The model under review builds one solid part; all positions refer to its coordinate system, in mm. A direction names the side the tool comes from. Coordinates: 2 decimals unless noted, no trailing zeros. Write each loop counter-clockwise with the first axis right and the second up, starting at its lowest first coordinate (ties: lowest second). Pieces come first, ordered by that corner, then holes. Notation, with made-up numbers: (-29.5, 71.5) - (-18.5, 71.5) arc R27 cw to (-18.5, 107.5) - close; hole circle Ø4 at (-32, 10). An arc over 180 degrees is marked (long way). Return JSON: item names as keys, results as strings. Group by question number.
(1) Draft analysis for pull direction X (two halves, no side actions). For faces 1 (the face through (-39.365, 61.689, -0.133)), 2 (the face through (61, -25, 61.925)), 3 (the face through (63.867, -25, 41)), 4 (the face through (114.667, -25, 52)), state which applies: released by +X, released by -X, zero draft, split by the parting line, or undercut.
(2) Tool access review of faces 5 (the face through (89, -25, 38.1)), 6 (the face through (68, -50.8, 45)), 7 (the face through (22.225, -33, 18)): name each direction out of +Z, -Z, +X, -X, +Y, -Y from which nothing blocks a thin tool from reaching the whole face with its end or side.
(3) To check wall thickness, follow L1, parallel to X at y = -31, z = -3 (3 decimals); L2, parallel to Z at x = 6, y = 33.5 (3 decimals); L3, parallel to Y at x = 89.5, z = 53.5. State the ranges of each line that lie inside material, in increasing order. Write a range as from..to.
(4) We need section B-B on z = -1.5. State the section outline as (x, y) points (3 decimals).
(5) For pin 1 Ø3 at (x, z) = (37.5, 41) entering from +Y; pin 2 Ø1 at (x, z) = (41.5, 24.5) entering from -Y; pin 3 Ø11 at (y, z) = (-4.5, 17) entering from +X (3 decimals); pin 4 Ø14 at (y, z) = (-28.5, 16) entering from -X (3 decimals), all flat-tipped, find the tip position at first contact; note any pin that passes through.
(6) We need section C-C on x = 76. State the section outline as (y, z) points (3 decimals), then the cut area to 3 significant figures.
(7) We need section A-A on y = -43.5. State the section outline as (x, z) points (3 decimals).
(8) We need section D-D on y = 43. State the section outline as (x, z) points (3 decimals), then the cut area to 3 significant figures.
```python
from build123d import *

# Parameters (mm, degrees)
F1_DEPTH = 63.5
F2_DEPTH = 50.8
F0_W     = 25.4
F0_H     = 19.05
F0_H_2   = 4.7498004709
F0_H_3   = 4.7751995291
F3_DEPTH = 50.8
F4_DEPTH = 15.875
F5_R     = 6.35


with BuildPart() as f1:
    # F0 (on Front) → F1 (new body, symmetric)
    with BuildSketch(Plane.XZ):
        Polygon((-41.275, 9.525), (-41.275, -9.525), (41.275, -9.525), (41.275, 9.525), (22.225, 9.525), align=None)
    extrude(amount=F1_DEPTH, both=True)

    # F0 (on Front) → F2 (join)
    with BuildSketch(Plane.XZ):
        with BuildLine():
            Line((22.225, 9.525), (41.275, 9.525))
            Line((41.275, 9.525), (41.275, 27.0002))
            ThreePointArc((41.275, 27.0002), (45.9246798487, 38.2255201513), (57.15, 42.8752))
            Line((57.15, 42.8752), (63.8665184379, 42.8752))
            Line((63.8665184379, 42.8752), (63.8665184379, 61.9252))
            Line((63.8665184379, 61.9252), (57.15, 61.9252))
            ThreePointArc((57.15, 61.9252), (32.4542956671, 51.6959043329), (22.225, 27.0002))
            Line((22.225, 27.0002), (22.225, 9.525))
        make_face()
    extrude(amount=F2_DEPTH)

    # F0 (on Front) → F3 (join)
    with BuildSketch(Plane.XZ):
        with Locations((76.5665184379, 52.4002)):
            Rectangle(F0_W, F0_H)
        Polygon((89.2665184379, 66.6750004709), (89.2665184379, 61.9252), (89.2665184379, 42.8752), (89.2665184379, 38.1000004709), (114.6665184379, 38.1000004709), (114.6665184379, 66.6750004709), align=None)
        with Locations((76.5665184379, 64.3001002354)):
            Rectangle(F0_W, F0_H_2)
        with Locations((76.5665184379, 40.4876002354)):
            Rectangle(F0_W, F0_H_3)
    extrude(amount=F3_DEPTH)

    # F0 (on Front) → F4 (join)
    with BuildSketch(Plane.XZ):
        Polygon((-41.275, 9.525), (-41.275, -9.525), (41.275, -9.525), (41.275, 9.525), (22.225, 9.525), align=None)
        with BuildLine():
            add(Edge.make_bspline(
                [(-41.275, 9.525), (-41.1059595644, 38.1653234363), (12.9924593493, 62.6207739115), (57.15, 61.9252)],
                knots=[0, 0, 0, 0, 111.5045361635, 111.5045361635, 111.5045361635, 111.5045361635], degree=3))
            Line((-41.275, 9.525), (22.225, 9.525))
            Line((22.225, 9.525), (22.225, 27.0002))
            ThreePointArc((22.225, 27.0002), (32.4542956671, 51.6959043329), (57.15, 61.9252))
        make_face()
        with BuildLine():
            Line((22.225, 9.525), (41.275, 9.525))
            Line((41.275, 9.525), (41.275, 27.0002))
            ThreePointArc((41.275, 27.0002), (45.9246798487, 38.2255201513), (57.15, 42.8752))
            Line((57.15, 42.8752), (63.8665184379, 42.8752))
            Line((63.8665184379, 42.8752), (63.8665184379, 61.9252))
            Line((63.8665184379, 61.9252), (57.15, 61.9252))
            ThreePointArc((57.15, 61.9252), (32.4542956671, 51.6959043329), (22.225, 27.0002))
            Line((22.225, 27.0002), (22.225, 9.525))
        make_face()
        with Locations((76.5665184379, 52.4002)):
            Rectangle(F0_W, F0_H)
        with Locations((76.5665184379, 64.3001002354)):
            Rectangle(F0_W, F0_H_2)
        with Locations((76.5665184379, 40.4876002354)):
            Rectangle(F0_W, F0_H_3)
        Polygon((89.2665184379, 66.6750004709), (89.2665184379, 61.9252), (89.2665184379, 42.8752), (89.2665184379, 38.1000004709), (114.6665184379, 38.1000004709), (114.6665184379, 66.6750004709), align=None)
    extrude(amount=F4_DEPTH)

    # F5
    f5_edges = [f1.edges().sort_by_distance(p)[0] for p in [
        (41.275, -63.5, 0),
        (-41.275, -63.5, 0),
        (41.275, 63.5, 0),
        (-41.275, 63.5, 0),
    ]]
    fillet(f5_edges, radius=F5_R)


solid = f1.part
```
Ans:
{
 "1": {"face 1": "released by -X", "face 2": "zero draft", "face 3": "undercut", "face 4": "released by +X"},
 "2": {"face 5": "-Z, +X, +Y, -Y", "face 6": "+Z, +X, -X, -Y", "face 7": "+Z, -X, -Y"},
 "3": {"L1": "-41.275..41.275", "L2": "-9.525..9.525", "L3": "-50.8..0"},
 "4": {"outline": "(-41.275, -57.15) arc R6.35 ccw to (-34.925, -63.5) - (34.925, -63.5) arc R6.35 ccw to (41.275, -57.15) - (41.275, 57.15) arc R6.35 ccw to (34.925, 63.5) - (-34.925, 63.5) arc R6.35 ccw to (-41.275, 57.15) - close"},
 "5": {"pin 1": "y = 0", "pin 2": "y = -50.8", "pin 3": "x = 41.275", "pin 4": "x = -41.275"},
 "6": {"outline": "(-50.8, 38.1) - (0, 38.1) - (0, 66.675) - (-50.8, 66.675) - close", "area": "1,450 mm²"},
 "7": {"outline": "(-41.275, -9.525) - (41.275, -9.525) - (41.275, 27) arc R15.875 cw to (57.15, 42.875) - (63.867, 42.875) - (63.867, 38.1) - (114.667, 38.1) - (114.667, 66.675) - (63.867, 66.675) - (63.867, 61.925) - (57.15, 61.925) arc R34.925 ccw to (22.225, 27) - (22.225, 9.525) - (-41.275, 9.525) - close"},
 "8": {"outline": "(-41.275, -9.525) - (41.275, -9.525) - (41.275, 9.525) - (-41.275, 9.525) - close", "area": "1,570 mm²"}
}
